```python
from build123d import *

# Parameters (mm, degrees)
F0_W = 15
F0_H = 40


with BuildPart() as f1:
    # F0 (on Front) → F1 (revolve)
    with BuildSketch(Plane.XZ):
        with Locations((0, 20)):
            Rectangle(F0_W, F0_H)
        Polygon((-25, 40), (-7.5, 40), (7.5, 40), (25, 40), (25, 45), (-25, 45), align=None)
    revolve(axis=Axis((0, 0, 0), (1, 0, 0)))


solid = f1.part
```
Could you check a few things on this model? Use its own coordinates, in mm. A direction names the side the tool comes from. Coordinates: 2 decimals unless noted, no trailing zeros. Write each loop counter-clockwise with the first axis right and the second up, starting at its lowest first coordinate (ties: lowest second). Pieces come first, ordered by that corner, then holes. Notation, with made-up numbers: (0.25, 3.5) -> (40.25, 3.5) arc R10 cw to (40.25, 9.5) -> close; hole circle Ø4 at (-4.5, 58). An arc over 180 degrees is marked (long way). Write item = value, one per line. Start each with the question number.
(1) Which directions (+Z, -Z, +X, -X, +Y, -Y) give clear straight access to the entire face, cutting with the end or side of a thin tool? Please do faces 1 (the face through (-25, 26.5, -30.2)), 2 (the face through (-7.5, -1, 1)), 3 (the face through (16.37, 39.05, -8.67)).
(2) I want a section at C-C (x = -4). Please give me the cut outline in (y, z), plus the area to 3 significant figures.
(3) I need wall thicknesses on line 1 (Y direction, x = 12, z = 0); line 2 (X direction, y = -7, z = -8). Which ranges of each line are inside material? Lowest first, please. Write a range as [from, to].
(4) I want a section at A-A (y = 0). Please give me the cut outline in (x, z), plus the area to 3 significant figures.
(5) We'd pull the mould along Z, two halves only. Please class faces 4 (the face through (-16.13, 39.05, -8.67)), 5 (the face through (-0.35, 39.923, 20.765)), 6 (the face through (25, 26.5, 30.2)): released by +Z, released by -Z, zero draft, split by the parting line, or undercut.
(6) Will these pins go through, and if not, where does the flat tip stop? pin 1 (3 mm diameter, centred on y = 21.5, z = -1, fed in from +X); pin 2 (1.5 mm diameter, centred on x = -0.5, z = 22, fed in from -Y); pin 3 (3 mm diameter, centred on x = -15, z = -14, fed in from +Y).
Result set:
q1.face_1 = +Z, -Z, -X, +Y, -Y
q1.face_2 = -X
q1.face_3 = +X
q2.outline = circle Ø90 at (0, 0)
q2.area = 6,360 mm2
q3.line_1 = [-45, -40], [40, 45]
q3.line_2 = [-7.5, 7.5]
q4.outline = (-25, -45) -> (25, -45) -> (25, -40) -> (7.5, -40) -> (7.5, 40) -> (25, 40) -> (25, 45) -> (-25, 45) -> (-25, 40) -> (-7.5, 40) -> (-7.5, -40) -> (-25, -40) -> close
q4.area = 1,700 mm2
q5.face_4 = undercut
q5.face_5 = split by the parting line
q5.face_6 = zero draft
q6.pin_1 = 7.5
q6.pin_2 = -39.67
q6.pin_3 = 43.23
